```python
from build123d import *

# Parameters (mm, degrees)
SKETCH_4_R      = 28.77
EXTRUDE_2_DEPTH = 3


with BuildPart() as part:
    # 草图4 → 凸台-拉伸2 (new body)
    with BuildSketch(Plane(origin=(0, 0, 0), x_dir=(1, 0, 0), z_dir=(0, 1, 0))):
        with BuildLine():
            Line((-10, 116.571866246), (-10, 136.571866246))
            Line((-10, 136.571866246), (10, 136.571866246))
            Line((10, 136.571866246), (10, 116.571866246))
            ThreePointArc((10, 116.571866246), (0, -117), (-10, 116.571866246))
        make_face()
        with Locations(Location((0, 0, 0), (0, 0, 270))):
            Circle(SKETCH_4_R, mode=Mode.SUBTRACT)
        with BuildLine():
            Line((-101.67701278, -47.156245315), (-97.293939129, -44.625676563))
            ThreePointArc((-97.293939129, -44.625676563), (-92.699359221, 53.52), (-10, 106.571861202))
            Line((-10, 106.571861202), (-10, 111.632998706))
            ThreePointArc((-10, 111.632998706), (-97.064127256, 56.04), (-101.67701278, -47.156245315))
        make_face(mode=Mode.SUBTRACT)
        with BuildLine():
            Line((-92.787212622, -42.023716801), (-88.138936726, -39.340033461))
            ThreePointArc((-88.138936726, -39.340033461), (-83.588771973, 48.26), (-10, 96.000574998))
            Line((-10, 96.000574998), (-10, 101.367941678))
            ThreePointArc((-10, 101.367941678), (-88.213347629, 50.93), (-92.787212622, -42.023716801))
        make_face(mode=Mode.SUBTRACT)
        with BuildLine():
            Line((-83.331028335, -36.564186257), (-78.318973499, -33.670475049))
            ThreePointArc((-78.318973499, -33.670475049), (-73.828665673, 42.625), (-10, 84.661458173))
            Line((-10, 84.661458173), (-10, 90.44888059))
            ThreePointArc((-10, 90.44888059), (-78.808311744, 45.5), (-83.331028335, -36.564186257))
        make_face(mode=Mode.SUBTRACT)
        with BuildLine():
            Line((-73.075202534, -30.64298247), (-67.527706459, -27.440134118))
            ThreePointArc((-67.527706459, -27.440134118), (-63.124591682, 36.445), (-10, 72.200776312))
            Line((-10, 72.200776312), (-10, 78.606473016))
            ThreePointArc((-10, 78.606473016), (-68.623852996, 39.62), (-73.075202534, -30.64298247))
        make_face(mode=Mode.SUBTRACT)
        with BuildLine():
            Line((-61.58540006, -24.009341919), (-55.118955246, -20.275938265))
            ThreePointArc((-55.118955246, -20.275938265), (-50.861671964, 29.365), (-10, 57.872384606))
            Line((-10, 57.872384606), (-10, 65.339191914))
            ThreePointArc((-10, 65.339191914), (-57.24427919, 33.05), (-61.58540006, -24.009341919))
        make_face(mode=Mode.SUBTRACT)
        with BuildLine():
            Line((-47.885927762, -16.0999479), (-39.407930409, -11.205173846))
            ThreePointArc((-39.407930409, -11.205173846), (-35.481060793, 20.485), (-10, 39.730855767))
            Line((-10, 39.730855767), (-10, 49.520403876))
            ThreePointArc((-10, 49.520403876), (-43.751603399, 25.26), (-47.885927762, -16.0999479))
        make_face(mode=Mode.SUBTRACT)
        with BuildLine():
            Line((-37.885927762, -33.420455976), (-29.407930409, -28.525681921))
            ThreePointArc((-29.407930409, -28.525681921), (0, -40.97), (29.407930409, -28.525681921))
            Line((29.407930409, -28.525681921), (37.885927762, -33.420455976))
            ThreePointArc((37.885927762, -33.420455976), (0, -50.52), (-37.885927762, -33.420455976))
        make_face(mode=Mode.SUBTRACT)
        with BuildLine():
            Line((-51.58540006, -41.329849995), (-45.118955246, -37.596446341))
            ThreePointArc((-45.118955246, -37.596446341), (0, -58.73), (45.118955246, -37.596446341))
            Line((45.118955246, -37.596446341), (51.58540006, -41.329849995))
            ThreePointArc((51.58540006, -41.329849995), (0, -66.1), (-51.58540006, -41.329849995))
        make_face(mode=Mode.SUBTRACT)
        with BuildLine():
            Line((-63.075202534, -47.963490546), (-57.527706459, -44.760642194))
            ThreePointArc((-57.527706459, -44.760642194), (0, -72.89), (57.527706459, -44.760642194))
            Line((57.527706459, -44.760642194), (63.075202534, -47.963490546))
            ThreePointArc((63.075202534, -47.963490546), (0, -79.24), (-63.075202534, -47.963490546))
        make_face(mode=Mode.SUBTRACT)
        with BuildLine():
            Line((-82.787212622, -59.344224877), (-78.138936726, -56.660541537))
            ThreePointArc((-78.138936726, -56.660541537), (0, -96.52), (78.138936726, -56.660541537))
            Line((78.138936726, -56.660541537), (82.787212622, -59.344224877))
            ThreePointArc((82.787212622, -59.344224877), (0, -101.86), (-82.787212622, -59.344224877))
        make_face(mode=Mode.SUBTRACT)
        with BuildLine():
            Line((-73.331028335, -53.884694333), (-68.318973499, -50.990983124))
            ThreePointArc((-68.318973499, -50.990983124), (0, -85.25), (68.318973499, -50.990983124))
            Line((68.318973499, -50.990983124), (73.331028335, -53.884694333))
            ThreePointArc((73.331028335, -53.884694333), (0, -91), (-73.331028335, -53.884694333))
        make_face(mode=Mode.SUBTRACT)
        with BuildLine():
            Line((-91.67701278, -64.476753391), (-87.293939129, -61.946184639))
            ThreePointArc((-87.293939129, -61.946184639), (0, -107.04), (87.293939129, -61.946184639))
            Line((87.293939129, -61.946184639), (91.67701278, -64.476753391))
            ThreePointArc((91.67701278, -64.476753391), (0, -112.08), (-91.67701278, -64.476753391))
        make_face(mode=Mode.SUBTRACT)
        with BuildLine():
            Line((10, 49.520403876), (10, 39.730855767))
            ThreePointArc((10, 39.730855767), (35.481060793, 20.485), (39.407930409, -11.205173846))
            Line((39.407930409, -11.205173846), (47.885927762, -16.0999479))
            ThreePointArc((47.885927762, -16.0999479), (43.751603399, 25.26), (10, 49.520403876))
        make_face(mode=Mode.SUBTRACT)
        with BuildLine():
            Line((10, 65.339191914), (10, 57.872384606))
            ThreePointArc((10, 57.872384606), (50.861671964, 29.365), (55.118955246, -20.275938265))
            Line((55.118955246, -20.275938265), (61.58540006, -24.009341919))
            ThreePointArc((61.58540006, -24.009341919), (57.24427919, 33.05), (10, 65.339191914))
        make_face(mode=Mode.SUBTRACT)
        with BuildLine():
            Line((10, 78.606473016), (10, 72.200776312))
            ThreePointArc((10, 72.200776312), (63.124591682, 36.445), (67.527706459, -27.440134118))
            Line((67.527706459, -27.440134118), (73.075202534, -30.64298247))
            ThreePointArc((73.075202534, -30.64298247), (68.623852996, 39.62), (10, 78.606473016))
        make_face(mode=Mode.SUBTRACT)
        with BuildLine():
            Line((10, 90.44888059), (10, 84.661458173))
            ThreePointArc((10, 84.661458173), (73.828665673, 42.625), (78.318973499, -33.670475049))
            Line((78.318973499, -33.670475049), (83.331028335, -36.564186257))
            ThreePointArc((83.331028335, -36.564186257), (78.808311744, 45.5), (10, 90.44888059))
        make_face(mode=Mode.SUBTRACT)
        with BuildLine():
            Line((10, 101.367941678), (10, 96.000574998))
            ThreePointArc((10, 96.000574998), (83.588771973, 48.26), (88.138936726, -39.340033461))
            Line((88.138936726, -39.340033461), (92.787212622, -42.023716801))
            ThreePointArc((92.787212622, -42.023716801), (88.213347629, 50.93), (10, 101.367941678))
        make_face(mode=Mode.SUBTRACT)
        with BuildLine():
            Line((10, 111.632998706), (10, 106.571861202))
            ThreePointArc((10, 106.571861202), (92.699359221, 53.52), (97.293939129, -44.625676563))
            Line((97.293939129, -44.625676563), (101.67701278, -47.156245315))
            ThreePointArc((101.67701278, -47.156245315), (97.064127256, 56.04), (10, 111.632998706))
        make_face(mode=Mode.SUBTRACT)
    extrude(amount=EXTRUDE_2_DEPTH)


solid = part.part
```
Check sheet for the modelled part. Datum: model origin and axes. Units: mm. A direction names the side the tool comes from. Round coordinates to 2 decimals unless told otherwise and drop trailing zeros. One line per item, written item: value. Start each with the question number.
Q1. Thickness scan on line 1 (X direction, y = 1.75, z = -122). Record the ranges inside material, lowest first.
Q2. Mould release check, pull along Z, two halves, no side actions. Record for faces 1 (the face through (5.004, 1.479, 116.893)), 2 (the face through (1.021, 1.479, 79.233)), 3 (the face through (28, 3, 17)): pulls with the +Z half, pulls with the -Z half, needs draft (parallel to the pull), parting line crosses it, or undercut.
Q3. Gauge pin test, flat ends, axial feed: pin 1 Ø1 at (y, z) = (2, 22) entering from +X; pin 2 Ø1.5 at (y, z) = (1.5, -74) entering from +X; pin 3 Ø0.9 at (y, z) = (2, -60.5) entering from +X. Record the tip position at first contact, or that the pin passes through.
Q4. Cross-section at A-A (x = 0). Give the number of separate pieces and of enclosed holes in the cut face, and give its area (3 significant figures).
Q5. Set-up check for faces 4 (the face through (28, 0, 17)), 5 (the face through (-51.218, 1.479, -28.739)): record each of +Z, -Z, +X, -X, +Y, -Y from which the full face is reachable in a straight line by a thin tool's end or side.
Completed:
1. line 1: x = -10 to 10
2. face 1: parting line crosses it
2. face 2: undercut
2. face 3: needs draft
3. pin 1: stops at x = 115.01
3. pin 2: stops at x = 91.23
3. pin 3: stops at x = 100.41
4. separate pieces: 8
4. enclosed holes: 0
4. area: 470 mm²
5. face 4: +Z, -Z, +X, -X, -Y
5. face 5: +Y, -Y
